from build123d import *

# Parameters (mm, degrees)
MAIN_DEPTH          = 17
CUT_EXTRUDE1_DEPTH  = 10
SKETCH3_R           = 1.5
CUT_EXTRUDE2_DEPTH  = 18
SKETCH4_W           = 2.9
SKETCH4_H           = 1
SKETCH4_W_2         = 1
SKETCH4_H_2         = 2.9
BOSS_EXTRUDE1_DEPTH = 7
SKETCH5_W           = 15
SKETCH5_H           = 2.9
BOSS_EXTRUDE2_DEPTH = 1
SKETCH6_R           = 1.5
CUT_EXTRUDE3_DEPTH  = 18
BOSS_EXTRUDE3_DEPTH = 15
SKETCH8_R           = 1.5
CUT_EXTRUDE4_DEPTH  = 18
SKETCH9_R           = 1.5
CUT_EXTRUDE5_DEPTH  = 18.67766953


with BuildPart() as part:
    # Sketch1 → Main (new body)
    with BuildSketch(Plane.XY):
        Polygon((-90, -90), (-72.32233047, -72.32233047), (-84.343145751, -60.30151519), (-97.04163056, -73), (-115, -73), (-115, -80), (-90, -80), align=None)
    extrude(amount=MAIN_DEPTH)

    # Sketch2 → Cut-Extrude1 (cut)
    with BuildSketch(Plane(origin=(-72.32233047, -72.32233047, 0), x_dir=(0.707106781, -0.707106781, 0), z_dir=(0.707106781, 0.707106781, 0))):
        Polygon((-3.55, -10), (0, -10), (0, 0), (-10, 0), (-10, -3.55), (-9, -3.55), (-9, -6.45), (-10, -6.45), (-10, -10), (-6.45, -10), (-6.45, -9), (-3.55, -9), align=None)
    extrude(amount=-CUT_EXTRUDE1_DEPTH, mode=Mode.SUBTRACT)

    # Sketch3 → Cut-Extrude2 (cut, through all)
    with BuildSketch(Plane.XY.offset(17)):
        with Locations((-79.393398282, -72.32233047)):
            Circle(SKETCH3_R)
    extrude(amount=-CUT_EXTRUDE2_DEPTH, mode=Mode.SUBTRACT)

    # Sketch4 → Boss-Extrude1 (add)
    with BuildSketch(Plane.XY.offset(10)):
        with Locations((-95, -80.5)):
            Rectangle(SKETCH4_W, SKETCH4_H)
        with Locations((-90.5, -85)):
            Rectangle(SKETCH4_W_2, SKETCH4_H_2)
    extrude(amount=BOSS_EXTRUDE1_DEPTH)

    # Sketch5 → Boss-Extrude2 (add)
    with BuildSketch(Plane.XZ.offset(80)):
        with Locations((-107.5, 5)):
            Rectangle(SKETCH5_W, SKETCH5_H)
    extrude(amount=BOSS_EXTRUDE2_DEPTH)

    # Sketch6 → Cut-Extrude3 (cut, through all)
    with BuildSketch(Plane(origin=(0, -73, 0), x_dir=(1, 0, 0), z_dir=(0, 1, 0))):
        with Locations((-110, -5)):
            Circle(SKETCH6_R)
    extrude(amount=-CUT_EXTRUDE3_DEPTH, mode=Mode.SUBTRACT)

    # Sketch7 → Boss-Extrude3 (add)
    with BuildSketch(Plane.ZY.offset(115)):
        Polygon((17, -80), (17, -90), (10, -90), (10, -86.45), (9, -86.45), (9, -83.55), (10, -83.55), (10, -80), align=None)
    extrude(amount=-BOSS_EXTRUDE3_DEPTH)

    # Sketch8 → Cut-Extrude4 (cut, through all)
    with BuildSketch(Plane.XY.offset(17)):
        with Locations((-110, -85)):
            Circle(SKETCH8_R)
    extrude(amount=-CUT_EXTRUDE4_DEPTH, mode=Mode.SUBTRACT)

    # Sketch9 → Cut-Extrude5 (cut, through all)
    with BuildSketch(Plane.ZY.offset(90)):
        with Locations((5, -85)):
            Circle(SKETCH9_R)
    extrude(amount=-CUT_EXTRUDE5_DEPTH, mode=Mode.SUBTRACT)


solid = part.part
Read the model definition and answer for the solid it produces. Units are mm, in the model's axes. A direction names the side the tool comes from. Round coordinates to 2 decimals unless told otherwise and drop trailing zeros. Write each loop counter-clockwise with the first axis right and the second up, starting at its lowest first coordinate (ties: lowest second). Pieces come first, ordered by that corner, then holes.
Q1. Flat-ended cylindrical pins translate along their axes: P1, Ø0.5, axis at x = -103.5, z = 9.5, coming from the +Y side; P2, Ø1.5, axis at y = -72, z = 6, coming from the -X side; P3, Ø0.5, axis at y = -80.5, z = 5, coming from the +X side. Find the tip coordinate at first contact, or state that the pin passes through.
Values:
P1: stops at y = -73
P2: stops at x = -96.79
P3: stops at x = -80.25
Q2. Find section C-C on z = 11. Determine the outline of the cut face in (x, y), and give its area (3 significant figures).
Values:
outline: (-115, -90) - (-100, -90) - (-100, -80) - (-96.45, -80) - (-96.45, -81) - (-93.55, -81) - (-93.55, -80) - (-90, -80) - (-90, -83.55) - (-91, -83.55) - (-91, -86.45) - (-90, -86.45) - (-90, -90) - (-72.32, -72.32) - (-84.34, -60.3) - (-97.04, -73) - (-115, -73) - close; hole circle Ø3 at (-110, -85); hole circle Ø3 at (-79.39, -72.32)
area: 622 mm2
Q3. Find section D-D on z = 7.75. Determine the outline of the cut face in (x, y).
Values:
outline: (-115, -80) - (-90, -80) - (-90, -90) - (-79.39, -79.39) - (-86.46, -72.32) - (-79.39, -65.25) - (-84.34, -60.3) - (-97.04, -73) - (-115, -73) - close
Q4. A tool of negligible diameter and unlimited length cuts with its end or side. For faces 1 (the face through (-104.9, -83.55, 9.5)), 2 (the face through (-105, -81, 5)), 3 (the face through (-82.5, -69.1, 3.55)), 4 (the face through (-108, -82, 10)), 5 (the face through (-104.9, -80.5, 6.45)), from which of +Z, -Z, +X, -X, +Y, -Y can it reach the whole face along a straight path? Write none if from no direction.
Values:
face 1: -Z, -X
face 2: -Z, -X, -Y
face 3: -Z, +X
face 4: -X
face 5: -X, -Y
Q5. Find section B-B on z = 5. Determine the outline of the cut face in (x, y).
Values:
outline: (-115, -81) - (-111.5, -81) - (-111.5, -73) - (-115, -73) - close; (-108.5, -81) - (-100, -81) - (-100, -80) - (-90, -80) - (-90, -83.5) - (-83.5, -83.5) - (-79.39, -79.39) - (-85.76, -73.03) - (-78.69, -65.96) - (-84.34, -60.3) - (-97.04, -73) - (-108.5, -73) - close; (-90, -90) - (-86.5, -86.5) - (-90, -86.5) - close
Q6. Find section A-A on y = -85.5. Determine the outline of the cut face in (x, z), and give its area (3 significant figures).
Values:
outline: (-115, 9) - (-111.41, 9) - (-111.41, 17) - (-115, 17) - close; (-108.59, 9) - (-100, 9) - (-100, 17) - (-108.59, 17) - close; (-91, 10) - (-90, 10) - (-90, 6.41) - (-85.5, 6.41) - (-85.5, 17) - (-91, 17) - close; (-90, 0) - (-85.5, 0) - (-85.5, 3.59) - (-90, 3.59) - close
area: 168 mm2
Q7. The mould has two halves that part along Y. Classify faces 6 (the face through (-104.9, -86.45, 9.5)), 7 (the face through (-87.518, -83.513, 4.805)), 8 (the face through (-105, -85, 9)): released by +Y, released by -Y, zero draft, split by the parting line, or undercut.
Values:
face 6: released by -Y
face 7: undercut
face 8: zero draft
Q8. Straight lines are drawn through the part: line 1 (Y direction, x = -110, z = 14); line 2 (Z direction, x = -88, y = -85); line 3 (Y direction, x = -82, z = 1.25). For each, find the intervals that lie inside material, in ascending order.
Values:
line 1: y = -90 to -86.5, -83.5 to -73
line 2: z = 0 to 3.5, 6.5 to 17
line 3: y = -82 to -76.79, -67.86 to -62.64
